The model under review builds one solid part; all positions refer to its coordinate system, in mm. Face numbers are marked on the shaded views. A direction names the side the tool comes from. Coordinates: 2 decimals unless noted, no trailing zeros. Write each loop counter-clockwise with the first axis right and the second up, starting at its lowest first coordinate (ties: lowest second). Pieces come first, ordered by that corner, then holes. Notation, with made-up numbers: (53.25, -10) - (93.25, -10) arc R24 ccw to (93.25, 29) - close; hole circle Ø6 at (-40, -40). An arc over 180 degrees is marked (long way). Return JSON: item names as keys, results as strings. Group by question number.
(1) We need section B-B on y = -71. State the section outline as (x, z) points.
(2) For pin 1 Ø3 at (y, z) = (-60, 4) entering from +X; pin 2 Ø5.5 at (y, z) = (-41.5, -3) entering from +X, all flat-tipped, find the tip position at first contact; note any pin that passes through.
(3) We need section C-C on z = 16. State the section outline as (x, y) points, then the cut area to 3 significant figures.
(4) To check wall thickness, follow L1, parallel to Y at x = 109, z = 22.5; L2, parallel to X at y = -78.5, z = 18.5; L3, parallel to X at y = -54, z = 41.5. State the ranges of each line that lie inside material, in increasing order. Write a range as from..to.
(5) We need section A-A on x = 261. State the section outline as (y, z) points, then the cut area to 3 significant figures.
(6) Draft analysis for pull direction Z (two halves, no side actions). For the marked faces 3, 4 and 5, state which applies: released by +Z, released by -Z, zero draft, split by the parting line, or undercut.
(7) Tool access review of the marked faces 1 and 2: name each direction out of +Z, -Z, +X, -X, +Y, -Y from which nothing blocks a thin tool from reaching the whole face with its end or side.
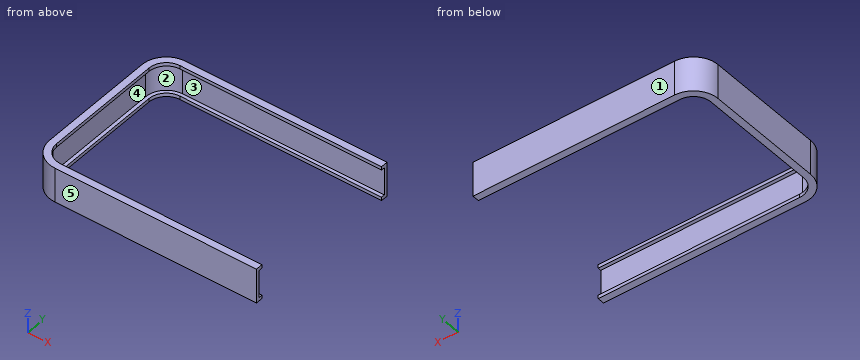
```python
from build123d import *

# Parameters (mm, degrees)
SALIENTE_EXTRUIR1_DEPTH = 40
SALIENTE_EXTRUIR2_DEPTH = 5
SALIENTE_EXTRUIR3_DEPTH = 290


with BuildPart() as part:
    # Croquis1 → Saliente-Extruir1 (new body)
    with BuildSketch(Plane.XY):
        with BuildLine():
            Line((-2.5, -85), (-2.5, 85))
            ThreePointArc((-2.5, 85), (7.751262658, 109.748737342), (32.5, 120))
            Line((32.5, 120), (32.5, 115))
            ThreePointArc((32.5, 115), (11.286796564, 106.213203436), (2.5, 85))
            Line((2.5, 85), (2.5, -85))
            ThreePointArc((2.5, -85), (11.286796564, -106.213203436), (32.5, -115))
            Line((32.5, -115), (32.5, -120))
            ThreePointArc((32.5, -120), (7.751262658, -109.748737342), (-2.5, -85))
        make_face()
    extrude(amount=SALIENTE_EXTRUIR1_DEPTH)

    # Croquis2 → Saliente-Extruir2 (add)
    with BuildSketch(Plane.XY.offset(40)):
        with BuildLine():
            Line((-2.5, 85), (-2.5, -85))
            ThreePointArc((-2.5, -85), (7.751262658, -109.748737342), (32.5, -120))
            Line((32.5, -120), (32.5, -110))
            ThreePointArc((32.5, -110), (14.82233047, -102.67766953), (7.5, -85))
            Line((7.5, -85), (7.5, 85))
            ThreePointArc((7.5, 85), (14.82233047, 102.67766953), (32.5, 110))
            Line((32.5, 110), (32.5, 120))
            ThreePointArc((32.5, 120), (7.751262658, 109.748737342), (-2.5, 85))
        make_face()
    saliente_extruir2 = extrude(amount=SALIENTE_EXTRUIR2_DEPTH)

    # Simetría1: Saliente-Extruir2 across plane
    add(saliente_extruir2.mirror(Plane.XY.offset(20)))

    # Croquis3 → Saliente-Extruir3 (add)
    with BuildSketch(Plane(origin=(32.5, 0, 0), x_dir=(0, 0, -1), z_dir=(1, 0, 0))):
        Polygon((-45, 120), (-45, 110), (-40, 110), (-40, 115), (0, 115), (0, 110), (5, 110), (5, 120), align=None)
        Polygon((-45, -110), (-40, -110), (-40, -115), (0, -115), (0, -110), (5, -110), (5, -120), (-45, -120), align=None)
    extrude(amount=SALIENTE_EXTRUIR3_DEPTH)


solid = part.part
```
Ans:
{
 "1": {"outline": "(-2.5, -5) - (7.5, -5) - (7.5, 0) - (2.5, 0) - (2.5, 40) - (7.5, 40) - (7.5, 45) - (-2.5, 45) - close"},
 "2": {"pin 1": "x = 2.5", "pin 2": "x = 7.5"},
 "3": {"outline": "(-2.5, -85) arc R35 ccw to (32.5, -120) - (322.5, -120) - (322.5, -115) - (32.5, -115) arc R30 cw to (2.5, -85) - (2.5, 85) arc R30 cw to (32.5, 115) - (322.5, 115) - (322.5, 120) - (32.5, 120) arc R35 ccw to (-2.5, 85) - close", "area": "4,260 mm²"},
 "4": {"L1": "-120..-115, 115..120", "L2": "-2.5..2.5", "L3": "-2.5..7.5"},
 "5": {"outline": "(-120, -5) - (-110, -5) - (-110, 0) - (-115, 0) - (-115, 40) - (-110, 40) - (-110, 45) - (-120, 45) - close; (110, -5) - (120, -5) - (120, 45) - (110, 45) - (110, 40) - (115, 40) - (115, 0) - (110, 0) - close", "area": "600 mm²"},
 "6": {"face 3": "undercut", "face 4": "undercut", "face 5": "zero draft"},
 "7": {"face 1": "+Z, -Z, +X, -X, +Y", "face 2": "+X"}
}
